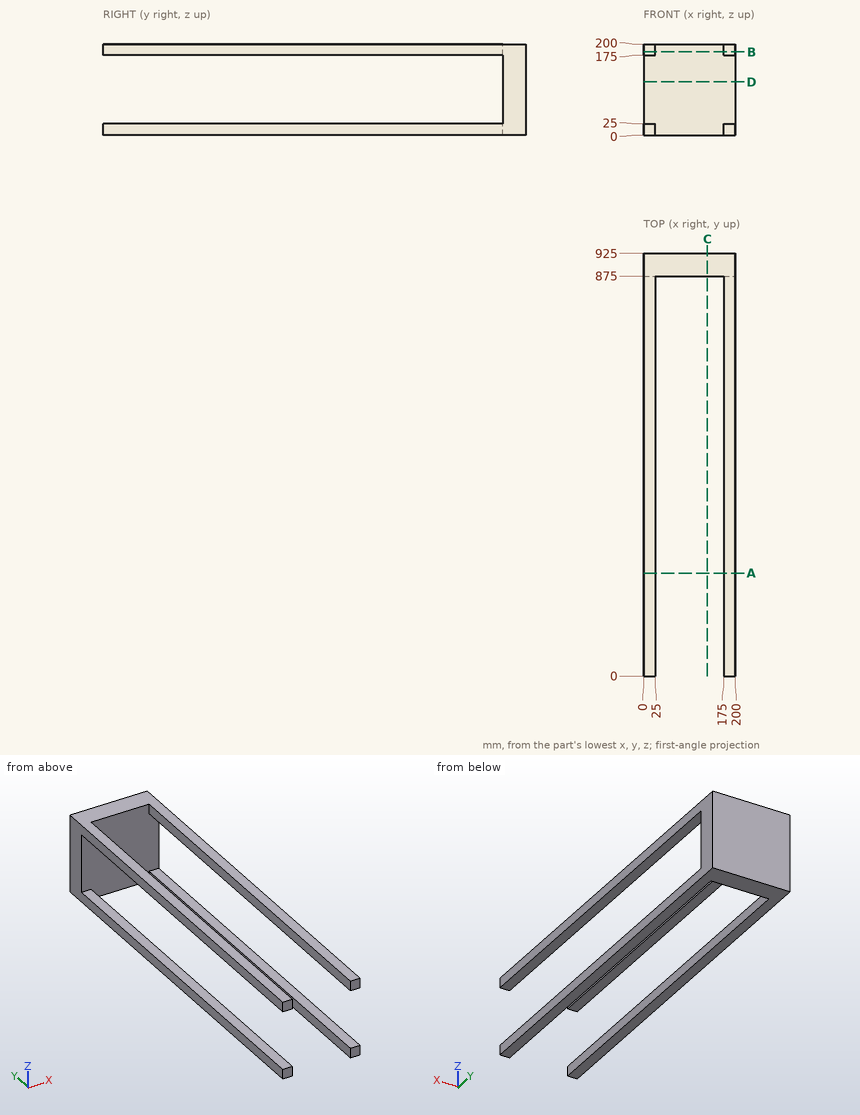
Could you check a few things on this drawing? It's one solid part, dimensions in mm from its lowest x, y, z. Give positions to 0.01 mm unless a question says otherwise; leave off trailing zeros. Write each loop counter-clockwise with the first axis right and the second up, starting at its lowest first coordinate (ties: lowest second). Pieces come first, ordered by that corner, then holes. Notation, with made-up numbers: (55, 1.25) -> (91, 1.25) arc R20 ccw to (91, 25.25) -> close; hole circle Ø10 at (-39, 48). An arc over 180 degrees is marked (long way). Answer as a JSON object with one key per item and string values.
Q1. Suppose I cut it at D-D on z = 117. Write out the boundary of the cut face in (x, y).
Taken from the geometry:
{"outline": "(0, 875) -> (200, 875) -> (200, 925) -> (0, 925) -> close"}
Q2. Suppose I cut it at C-C on x = 139.5. Write out the boundary of the cut face in (y, z), then the cut area to 3 significant figures.
Taken from the geometry:
{"outline": "(875, 0) -> (925, 0) -> (925, 200) -> (875, 200) -> close", "area": "10,000 mm²"}
Q3. Suppose I cut it at A-A on y = 225. Write out the boundary of the cut face in (x, z).
Taken from the geometry:
{"outline": "(0, 0) -> (25, 0) -> (25, 25) -> (0, 25) -> close; (0, 175) -> (25, 175) -> (25, 200) -> (0, 200) -> close; (175, 0) -> (200, 0) -> (200, 25) -> (175, 25) -> close; (175, 175) -> (200, 175) -> (200, 200) -> (175, 200) -> close"}
Q4. Suppose I cut it at B-B on z = 183. Write out the boundary of the cut face in (x, y).
Taken from the geometry:
{"outline": "(0, 0) -> (25, 0) -> (25, 875) -> (175, 875) -> (175, 0) -> (200, 0) -> (200, 925) -> (0, 925) -> close"}
Q5. Will this pin go through, and if not, where does the flat tip stop? pin 1 Ø12 at (x, z) = (118, 174) entering from -Y.
Taken from the geometry:
{"pin 1": "stops at y = 875"}
Q6. Please list where these lines run through material, in increasing order: L1, parallel to Z at x = 19, y = 68; L2, parallel to Y at x = 93.5, z = 142.
Taken from the geometry:
{"L1": "z = 0 to 25, 175 to 200", "L2": "y = 875 to 925"}
